```python
from build123d import *

# Parameters (mm, degrees)
BOSS_EXTRUDE1_DEPTH            = 1.6
SKETCH2_R                      = 1.5
CUT_EXTRUDE1_DEPTH             = 68.287145875
CUT_EXTRUDE4_REACH             = 69.287
SKETCH3_W                      = 5
SKETCH3_H                      = 100
CUT_EXTRUDE4_DIRECTION_2_DEPTH = 68.287145875


with BuildPart() as part:
    # Sketch1 → Boss-Extrude1 (new body)
    with BuildSketch(Plane(origin=(0, 0, 0), x_dir=(1, 0, 0), z_dir=(0, 1, 0))):
        with BuildLine():
            Line((-13.938774234, 50), (13.938774234, 50))
            ThreePointArc((13.938774234, 50), (35.432285481, 41.173831077), (45, 20))
            Line((45, 20), (35, 20))
            Line((35, 20), (35, -40))
            Line((35, -40), (45, -40))
            Line((45, -40), (45, -41))
            ThreePointArc((45, -41), (42.363961031, -47.363961031), (36, -50))
            Line((36, -50), (-36, -50))
            ThreePointArc((-36, -50), (-42.363961031, -47.363961031), (-45, -41))
            Line((-45, -41), (-45, -40))
            Line((-45, -40), (-35, -40))
            Line((-35, -40), (-35, 20))
            Line((-35, 20), (-45, 20))
            ThreePointArc((-45, 20), (-35.432285481, 41.173831077), (-13.938774234, 50))
        make_face()
    extrude(amount=BOSS_EXTRUDE1_DEPTH)

    # Sketch2 → Cut-Extrude1 (cut, through all)
    with BuildSketch(Plane(origin=(0, 1.6, 0), x_dir=(1, 0, 0), z_dir=(0, 1, 0))):
        with Locations(Location((-26.5, 3, 0), (0, 0, 270))):
            Circle(SKETCH2_R)
        with Locations(Location((-26.5, -23, 0), (0, 0, 270))):
            Circle(SKETCH2_R)
        with Locations(Location((26.5, -23, 0), (0, 0, 90))):
            Circle(SKETCH2_R)
        with Locations(Location((26.5, 3, 0), (0, 0, 90))):
            Circle(SKETCH2_R)
    extrude(amount=-CUT_EXTRUDE1_DEPTH, mode=Mode.SUBTRACT)

    # Sketch3 → Cut-Extrude4 (cut, up to next)
    with BuildSketch(Plane(origin=(0, 0, 0), x_dir=(1, 0, 0), z_dir=(0, 1, 0)), mode=Mode.PRIVATE) as cut_extrude4_sk1:
        Rectangle(SKETCH3_W, SKETCH3_H)
    cut_extrude4_tool1 = extrude(cut_extrude4_sk1.sketch, amount=CUT_EXTRUDE4_REACH, mode=Mode.PRIVATE) & part.part
    add(cut_extrude4_tool1.solids().sort_by_distance((0, 0, 0))[0], mode=Mode.SUBTRACT)

    # Sketch3 → Cut-Extrude4 direction 2 (cut)
    with BuildSketch(Plane(origin=(0, 0, 0), x_dir=(1, 0, 0), z_dir=(0, 1, 0))):
        Rectangle(SKETCH3_W, SKETCH3_H)
    extrude(amount=-CUT_EXTRUDE4_DIRECTION_2_DEPTH, mode=Mode.SUBTRACT)


with BuildPart() as cut_extrude4_piece_1:
    # of the separate pieces the step leaves, piece 1, a body of its own (cut_extrude4_pieces)
    add(part.part.solids().sort_by_distance((2.5, 0, -50))[0])


with BuildPart() as cut_extrude4_piece_2:
    # of the separate pieces the step leaves, piece 2, a body of its own (cut_extrude4_pieces)
    add(part.part.solids().sort_by_distance((-45, 0, -20))[0])


with BuildPart() as cut_extrude4_piece_2_1:
    # Body-Move/Copy1: moved
    add(cut_extrude4_piece_2.part.moved(Location((5, 0, 0))))


with BuildPart() as cut_extrude4_piece_1_1:
    add(cut_extrude4_piece_1.part)

    # Combine1: union Cut-Extrude4 piece 2
    add(cut_extrude4_piece_2_1.part)


solid = cut_extrude4_piece_1_1.part
```
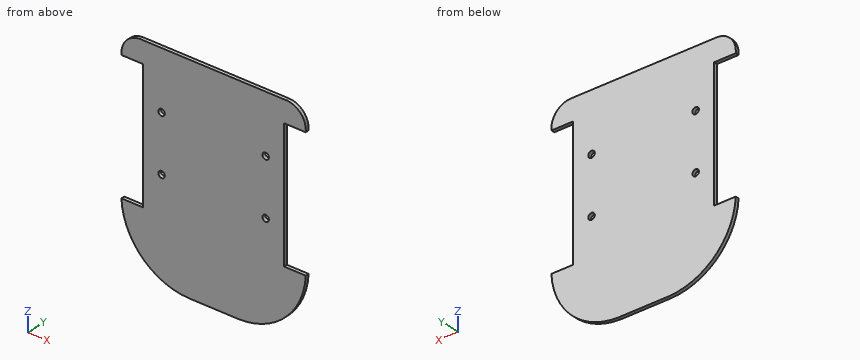
CAD build for the part. Positions are in the model's coordinates, mm. Round coordinates to 2 decimals unless told otherwise and drop trailing zeros. Loops run counter-clockwise (first coordinate to the right, second up) from the corner with the lowest first, then second, coordinate; pieces in that order, holes last. Notation, with made-up numbers: (5.5, -24.75) - (60.5, -24.75) arc R21 cw to (60.5, -14.75) - close; hole circle Ø8 at (68.5, 56). An arc over 180 degrees is marked (long way). Return JSON: item names as keys, results as strings. Group by question number.
Q1. Band-saw the part on A-A on y = 1.05. Give the cut face in (x, z).
Q2. Flat gauge pins, fed straight in: pin 1 Ø0.5 at (y, z) = (0.5, 11) entering from -X; pin 2 Ø2.5 at (x, z) = (26.5, 23) entering from +Y; pin 3 Ø0.8 at (x, y) = (39, 1) entering from +Z. Where does each tip first touch, or does it go through?
Q3. Band-saw the part on C-C on x = -21.5. Give the cut face in (y, z).
Q4. Band-saw the part on D-D on z = -6.5. Give the cut face in (x, y), plus the area to 3 significant figures.
Q5. Drill centre lines: line 1 along X through (y, z) = (0.3, 23); line 2 along Z through (x, y) = (26, 0.95); line 3 along Z through (x, y) = (26.5, 1.2). Where is each one in solid material? Low to high. Write a range as [from, to].
Q6. Band-saw the part on B-B on z = 23. Give the cut face in (x, y).
Solutions:
{
 "1": {"outline": "(-40, -20) arc R31.45 ccw to (-8.94, -50) - (13.94, -50) arc R31.45 ccw to (45, -20) - (35, -20) - (35, 40) - (45, 40) - (45, 41) arc R9 ccw to (36, 50) - (-31, 50) arc R9 ccw to (-40, 41) - (-40, 40) - (-30, 40) - (-30, -20) - close; hole circle Ø3 at (-21.5, -3); hole circle Ø3 at (-21.5, 23); hole circle Ø3 at (26.5, -3); hole circle Ø3 at (26.5, 23)"},
 "2": {"pin 1": "stops at x = -30", "pin 2": "passes through", "pin 3": "stops at z = 49.62"},
 "3": {"outline": "(0, -47.23) - (1.6, -47.23) - (1.6, -4.5) - (0, -4.5) - close; (0, -1.5) - (1.6, -1.5) - (1.6, 21.5) - (0, 21.5) - close; (0, 24.5) - (1.6, 24.5) - (1.6, 50) - (0, 50) - close"},
 "4": {"outline": "(-30, 0) - (35, 0) - (35, 1.6) - (-30, 1.6) - close", "area": "104 mm^2"},
 "5": {"line 1": "x = [-30, -23], [-20, 25], [28, 35]", "line 2": "z = [-47.45, -4.41], [-1.59, 21.59], [24.41, 50]", "line 3": "z = [-47.23, -4.5], [-1.5, 21.5], [24.5, 50]"},
 "6": {"outline": "(-30, 0) - (-23, 0) - (-23, 1.6) - (-30, 1.6) - close; (-20, 0) - (25, 0) - (25, 1.6) - (-20, 1.6) - close; (28, 0) - (35, 0) - (35, 1.6) - (28, 1.6) - close"}
}
